For this review, use the dimensioned drawing (mm, ordinates from the lowest corner) and the shaded views. Give positions to 0.01 mm unless a question says otherwise; leave off trailing zeros. Order: outer loops, then holes, each group sorted by start corner. A loop starts at its lowest first (then second) coordinate and runs counter-clockwise, first axis right, second up.
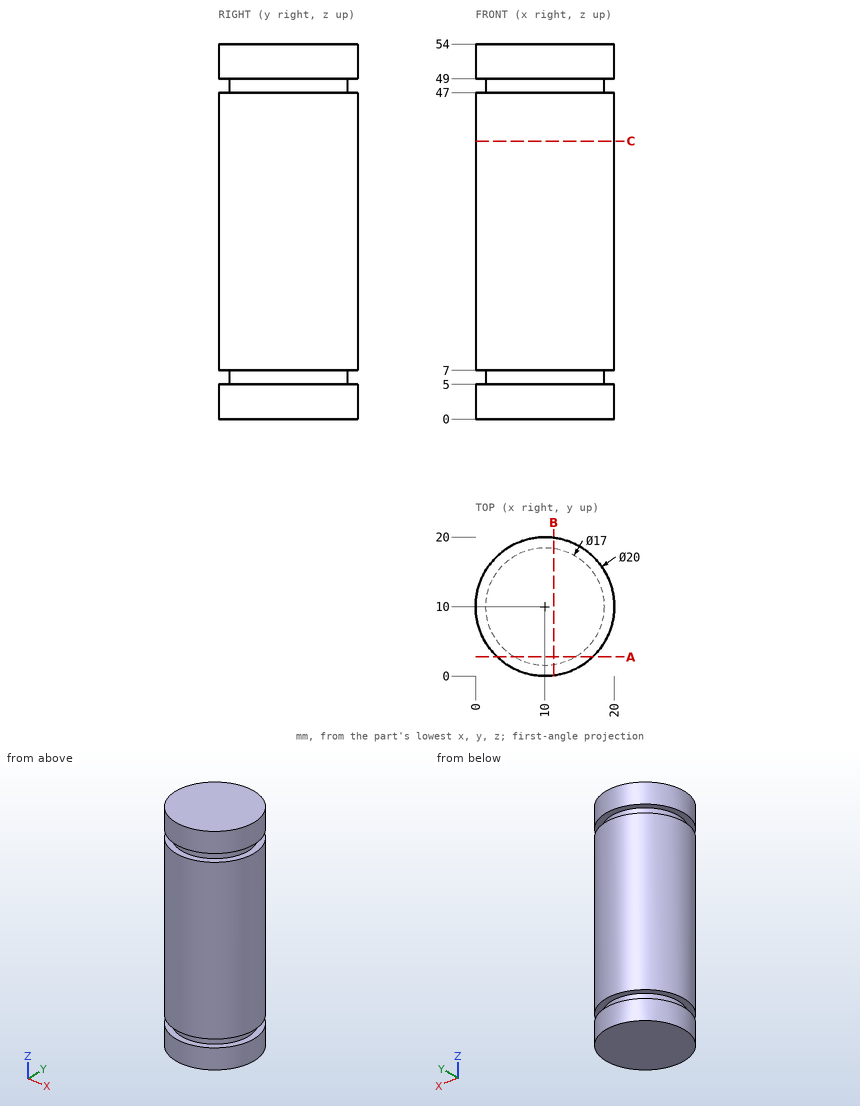
1. Take a section at C-C (z = 40). State the section outline as (x, y) points, then the cut area to 3 significant figures.
Recorded:
outline: circle Ø20 at (10, 10)
area: 314 mm2
2. Take a section at B-B (x = 11.25). State the section outline as (y, z) points, then the cut area to 3 significant figures.
Recorded:
outline: (0.08, 0) - (19.92, 0) - (19.92, 5) - (18.41, 5) - (18.41, 7) - (19.92, 7) - (19.92, 47) - (18.41, 47) - (18.41, 49) - (19.92, 49) - (19.92, 54) - (0.08, 54) - (0.08, 49) - (1.59, 49) - (1.59, 47) - (0.08, 47) - (0.08, 7) - (1.59, 7) - (1.59, 5) - (0.08, 5) - close
area: 1,060 mm2
3. For line 1 along Z through (x, y) = (17.5, 16.5); line 2 along X through (y, z) = (4.75, 13.5); line 3 along X through (y, z) = (9.75, 4.5), list the stretches that pass through material, from the lowest coordinate up.
Recorded:
line 1: z = 0 to 5, 7 to 47, 49 to 54
line 2: x = 1.49 to 18.51
line 3: x = 0 to 20
4. Take a section at A-A (y = 2.75). State the section outline as (x, z) points, then the cut area to 3 significant figures.
Recorded:
outline: (3.11, 0) - (16.89, 0) - (16.89, 5) - (14.44, 5) - (14.44, 7) - (16.89, 7) - (16.89, 47) - (14.44, 47) - (14.44, 49) - (16.89, 49) - (16.89, 54) - (3.11, 54) - (3.11, 49) - (5.56, 49) - (5.56, 47) - (3.11, 47) - (3.11, 7) - (5.56, 7) - (5.56, 5) - (3.11, 5) - close
area: 724 mm2
5. For pin 1 (1.5 mm diameter, centred on y = 17, z = 19.5, fed in from -X); pin 2 (6 mm diameter, centred on x = 14, z = 43, fed in from +Y), all flat-tipped, find the tip position at first contact; note any pin that passes through.
Recorded:
pin 1: stops at x = 2.19
pin 2: stops at y = 19.95
